For this review, take the finished solid that the model builds, in its own axes (mm). A direction names the side the tool comes from. Give positions to 0.01 mm unless a question says otherwise; leave off trailing zeros. Loops run counter-clockwise (first coordinate to the right, second up) from the corner with the lowest first, then second, coordinate; pieces in that order, holes last. Notation, with made-up numbers: (43, -31) - (102, -31) arc R23 cw to (102, -21) - close; hole circle Ø8 at (-30.75, 0.5). An arc over 180 degrees is marked (long way). Answer in a Markdown table with one row per item.
```python
from build123d import *

# Parameters (mm, degrees)
SKETCH1_R           = 25.6
BOSS_EXTRUDE1_DEPTH = 15
SKETCH2_R           = 3.15
CUT_EXTRUDE1_DEPTH  = 30
SKETCH3_R           = 7
CUT_EXTRUDE2_DEPTH  = 6
SKETCH4_R           = 3.15
CUT_EXTRUDE3_DEPTH  = 93.660671285
FILLET1_R           = 7
CHAMFER1_SIZE       = 0.5
CUT_EXTRUDE4_DEPTH  = 33


with BuildPart() as part:
    # Sketch1 → Boss-Extrude1 (new, symmetric)
    with BuildSketch(Plane(origin=(0, 0, 0), x_dir=(1, 0, 0), z_dir=(0, 1, 0))):
        with BuildLine():
            Line((-33.986502727, 0.957931299), (-35, -35))
            Line((-35, -35), (-60, -35))
            Line((-60, -35), (-60, -45))
            Line((-60, -45), (60, -45))
            Line((60, -45), (60, -35))
            Line((60, -35), (35, -35))
            Line((35, -35), (33.986502727, 0.957931299))
            ThreePointArc((33.986502727, 0.957931299), (0, 34), (-33.986502727, 0.957931299))
        make_face()
        with Locations(Location((0, 0, 0), (0, 0, 270))):
            Circle(SKETCH1_R, mode=Mode.SUBTRACT)
    extrude(amount=BOSS_EXTRUDE1_DEPTH, both=True)

    # Sketch2 → Cut-Extrude1 (cut)
    with BuildSketch(Plane.XY.offset(45)):
        Circle(SKETCH2_R)
    extrude(amount=-CUT_EXTRUDE1_DEPTH, mode=Mode.SUBTRACT)

    # Sketch3 → Cut-Extrude2 (cut)
    with BuildSketch(Plane.XY.offset(45)):
        Circle(SKETCH3_R)
    extrude(amount=-CUT_EXTRUDE2_DEPTH, mode=Mode.SUBTRACT)

    # Sketch4 → Cut-Extrude3 (cut, through all)
    with BuildSketch(Plane(origin=(0, 0, 35), x_dir=(-1, 0, 0), z_dir=(0, 0, -1))):
        with Locations((-50, 0)):
            Circle(SKETCH4_R)
        with Locations((50, 0)):
            Circle(SKETCH4_R)
    extrude(amount=-CUT_EXTRUDE3_DEPTH, mode=Mode.SUBTRACT)

    # Fillet1
    fillet1_edges = [part.edges().sort_by_distance(p)[0] for p in [
        (-35, 0, 35),
        (35, 0, 35),
    ]]
    fillet(fillet1_edges, radius=FILLET1_R)

    # Chamfer1
    chamfer1_edges = [part.edges().sort_by_distance(p)[0] for p in [
        (-34.397381029, -15, 13.619644926),
        (0, -15, -34),
        (50.90274024, -15, 35),
        (0, 15, -34),
        (60, 0, 35),
        (-60, 0, 35),
        (-34.397381029, 15, 13.619644926),
        (0, -15, -25.6),
        (0, 15, -25.6),
        (-60, 15, 40),
        (0, 15, 45),
        (60, 15, 40),
        (53.15, 0, 35),
        (-46.85, 0, 35),
        (50.90274024, 15, 35),
        (-50.90274024, -15, 35),
        (-50.90274024, 15, 35),
        (34.397381029, -15, 13.619644926),
        (34.397381029, 15, 13.619644926),
        (-36.9259594, -15, 33.018991335),
        (-36.9259594, 15, 33.018991335),
        (36.9259594, -15, 33.018991335),
        (36.9259594, 15, 33.018991335),
        (60, -15, 40),
        (0, -15, 45),
        (-60, -15, 40),
    ]]
    chamfer(chamfer1_edges, length=CHAMFER1_SIZE)

    # Sketch5 → Cut-Extrude4 (cut)
    with BuildSketch(Plane.XY):
        Polygon((2.944486373, 5.1), (-2.944486373, 5.1), (-5.888972746, 0), (-2.944486373, -5.1), (2.944486373, -5.1), (5.888972746, 0), align=None)
    extrude(amount=CUT_EXTRUDE4_DEPTH, mode=Mode.SUBTRACT)


solid = part.part
```
1. Clearance check with flat-ended pins moving along their axes: pin 1 (7 mm diameter, centred on x = -2.5, y = -0.5, fed in from +Z); pin 2 (7 mm diameter, centred on x = 50, y = 0, fed in from -Z); pin 3 (14 mm diameter, centred on x = -46.5, y = -0.5, fed in from -Z). State where each tip first meets the part, or that it passes through.
Values:
| item | result |
|---|---|
| pin 1 | stops at z = 39 |
| pin 2 | stops at z = 35.15 |
| pin 3 | stops at z = 34.61 |
2. Mouldability with a two-part tool opening along Y and no side actions: class faces 1 (the face through (-2.5, -1.917, 36.042)), 2 (the face through (-36.772, 14.642, 33.067)), 3 (the face through (0, -5.1, 29)), 4 (the face through (0.734, 0.203, -33.992)) as released by +Y, released by -Y, zero draft, split by the parting line, or undercut.
Values:
| item | result |
|---|---|
| face 1 | undercut |
| face 2 | released by +Y |
| face 3 | undercut |
| face 4 | zero draft |
3. We need section A-A, the plane x = 50. Give the boundary of the cut face in (y, z).
Values:
| item | result |
|---|---|
| outline | (-15, 35.5) - (-14.5, 35) - (-3.65, 35) - (-3.15, 35.5) - (-3.15, 45) - (-14.5, 45) - (-15, 44.5) - close; (3.15, 35.5) - (3.65, 35) - (14.5, 35) - (15, 35.5) - (15, 44.5) - (14.5, 45) - (3.15, 45) - close |
4. We need section B-B, the plane x = 0. Give the boundary of the cut face in (y, z).
Values:
| item | result |
|---|---|
| outline | (-15, -33.5) - (-14.5, -34) - (14.5, -34) - (15, -33.5) - (15, -26.1) - (14.5, -25.6) - (-14.5, -25.6) - (-15, -26.1) - close; (-15, 26.1) - (-14.5, 25.6) - (-5.1, 25.6) - (-5.1, 33) - (-3.15, 33) - (-3.15, 39) - (-7, 39) - (-7, 45) - (-14.5, 45) - (-15, 44.5) - close; (3.15, 33) - (5.1, 33) - (5.1, 25.6) - (14.5, 25.6) - (15, 26.1) - (15, 44.5) - (14.5, 45) - (7, 45) - (7, 39) - (3.15, 39) - close |
5. We need section C-C, the plane y = -8.5. Give the boundary of the cut face in (x, z), and give its area (3 significant figures).
Values:
| item | result |
|---|---|
| outline | (-60, 35.5) - (-59.5, 35) - (-41.81, 35) arc R7 cw to (-34.81, 28.2) - (-33.99, -0.96) arc R34 ccw to (33.99, -0.96) - (34.81, 28.2) arc R7 cw to (41.81, 35) - (59.5, 35) - (60, 35.5) - (60, 45) - (-60, 45) - close; hole circle Ø51.2 at (0, 0) |
| area | 3,390 mm^2 |
6. For faces 5 (the face through (53, 3, 35)), 6 (the face through (6.466, -2.681, 42.042)), 7 (the face through (-52.5, 3.4, 35)), 8 (the face through (0, -15, 28)), 9 (the face through (3, 2, 33)), list the 3-axis set-ups (+Z, -Z, +X, -X, +Y, -Y) from which the entire face can be reached by the end or side of a thin tool; tool diameter is ignored.
Values:
| item | result |
|---|---|
| face 5 | -Z, +X, +Y, -Y |
| face 6 | +Z |
| face 7 | -Z, -X, +Y, -Y |
| face 8 | +Z, -Z, +X, -X, -Y |
| face 9 | none |
7. Wall thickness on line 1 (Y direction, x = 0, z = 40); line 2 (Z direction, x = -0.5, y = 14); line 3 (Z direction, x = -1, y = 5.5): over which ranges is each line inside the solid? List them lowest first. Write a range as [from, to].
Values:
| item | result |
|---|---|
| line 1 | y = [-15, -7], [7, 15] |
| line 2 | z = [-34, -25.6], [25.6, 45] |
| line 3 | z = [-33.99, -25.58], [25.58, 39] |
